Verification items for the finished model (mm, model axes). Give positions to 0.01 mm unless a question says otherwise; leave off trailing zeros. Order: outer loops, then holes, each group sorted by start corner. A loop starts at its lowest first (then second) coordinate and runs counter-clockwise, first axis right, second up. Notation, with made-up numbers: M -17.75,-23.5 L -0.75,-23.5 A18 ccw -0.75,9.5 Z; hole C 83.5,24 d5. An arc over 180 degrees is marked long. Answer as a JSON object with one key per item and string values.
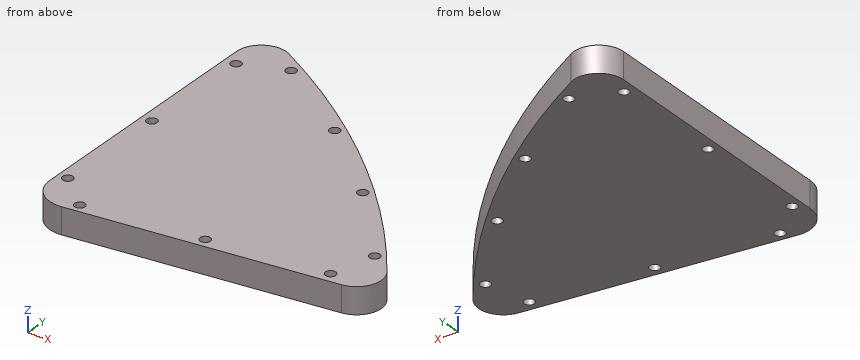
```python
from build123d import *

# Parameters (mm, degrees)
BOSS_EXTRUDE1_DEPTH = 12.7
SKETCH2_R           = 2.5
CUT_EXTRUDE1_DEPTH  = 188.024650501


with BuildPart() as part:
    # Sketch1 → Boss-Extrude1 (new body)
    with BuildSketch(Plane.XY):
        with BuildLine():
            Line((0.928877391, -25.603544091), (126.263071952, -11.506498815))
            ThreePointArc((126.263071952, -11.506498815), (135.842076702, -4.482224693), (134.616347537, 7.332822786))
            ThreePointArc((134.616347537, 7.332822786), (74.665711789, 73.710136722), (1.625549575, 125.335336338))
            ThreePointArc((1.625549575, 125.335336338), (-10.25140355, 125.146277033), (-16.085786649, 114.799406357))
            Line((-16.085786649, 114.799406357), (-15.166957214, -11.321736852))
            ThreePointArc((-15.166957214, -11.321736852), (-10.298375042, -22.045804112), (0.928877391, -25.603544091))
        make_face()
    extrude(amount=BOSS_EXTRUDE1_DEPTH)

    # Sketch2 → Cut-Extrude1 (cut, through all)
    with BuildSketch(Plane(origin=(0, 0, 0), x_dir=(-1, 0, 0), z_dir=(0, 0, -1))):
        with Locations((10.480661871, 106.771257069)):
            Circle(SKETCH2_R)
        with Locations((10.480661871, 50.510257069)):
            Circle(SKETCH2_R)
        with Locations((10.480661871, -5.750742931)):
            Circle(SKETCH2_R)
        with Locations((-52.065748574, 86.409889957)):
            Circle(SKETCH2_R)
        with Locations(Location((-89.964774668, 52.78214722, 0), (0, 0, 180))):
            Circle(SKETCH2_R)
        with Locations(Location((-123.32009462, 14.643139741, 0), (0, 0, 180))):
            Circle(SKETCH2_R)
        with Locations((-10.228252117, 114.989343254)):
            Circle(SKETCH2_R)
        with Locations(Location((-117.624924608, -6.89661647, 0), (0, 0, 180))):
            Circle(SKETCH2_R)
        with Locations(Location((-61.763750637, -13.592089836, 0), (0, 0, 180))):
            Circle(SKETCH2_R)
        with Locations(Location((-5.902576666, -20.287563201, 0), (0, 0, 180))):
            Circle(SKETCH2_R)
    extrude(amount=-CUT_EXTRUDE1_DEPTH, mode=Mode.SUBTRACT)


solid = part.part
```
Q1. Section check C-C on x = 19.5. Record the cut outline in (y, z).
Resolved:
{"outline": "M -23.51,0 L 114.85,0 L 114.85,12.7 L -23.51,12.7 Z"}
Q2. Gauge pin test, flat ends, axial feed: pin 1 Ø6 at (x, z) = (13.5, 10.5) entering from +Y; pin 2 Ø6 at (x, y) = (-10.48, 50.51) entering from -Z; pin 3 Ø5 at (y, z) = (40, 4.5) entering from -X; pin 4 Ø3 at (y, z) = (90, 7.5) entering from -X. Record the tip position at first contact, or that the pin passes through.
Resolved:
{"pin 1": "stops at y = 120.28", "pin 2": "stops at z = 0", "pin 3": "stops at x = -15.56", "pin 4": "stops at x = -15.92"}
Q3. Section check A-A on z = 3.5. Count the separate pieces of the cut face and the enclosed holes in it, then the cut area to 3 significant figures.
Resolved:
{"separate pieces": "1", "enclosed holes": "10", "area": "14,800 mm²"}
Q4. Section check B-B on y = 31.5. Record the cut outline in (x, z).
Resolved:
{"outline": "M -15.48,0 L 115.79,0 L 115.79,12.7 L -15.48,12.7 Z"}
Q5. Material ranges on L1, parallel to X at y = -6, z = 4.75; L2, parallel to Y at x = 64, z = 4.5; L3, parallel to Y at x = 88, z = 1.5, recorded low to high.
Resolved:
{"L1": "x = -15.21 to -12.97, -7.99 to 115.29, 119.96 to 135.03", "L2": "y = -18.51 to -14.71, -12.47 to 82.85", "L3": "y = -15.81 to 51.24, 54.33 to 61.33"}
